```python
from build123d import *

# Parameters (mm, degrees)
SKETCH_1_R          = 18.5
EXTRUDE_1_DEPTH     = 33
SKETCH_2_R          = 18
EXTRUDE_2_DEPTH     = 50
SKETCH_3_R          = 1.6
CUT_EXTRUDE_1_DEPTH = 6
SKETCH_4_R          = 6
EXTRUDE_3_DEPTH     = 6
SKETCH_5_R          = 3
EXTRUDE_4_DEPTH     = 15
CUT_EXTRUDE_START   = -12
CUT_EXTRUDE_2_DEPTH = 12


with BuildPart() as part:
    # 草图1 → 凸台-拉伸1 (new body)
    with BuildSketch(Plane.XY):
        Circle(SKETCH_1_R)
    extrude(amount=EXTRUDE_1_DEPTH)

    # 草图2 → 凸台-拉伸2 (add)
    with BuildSketch(Plane(origin=(0, 0, 0), x_dir=(-1, 0, 0), z_dir=(0, 0, -1))):
        Circle(SKETCH_2_R)
    extrude(amount=EXTRUDE_2_DEPTH)

    # 草图3 → 切除-拉伸1 (cut)
    with BuildSketch(Plane.XY.offset(33)):
        with Locations((-15.5, 0)):
            Circle(SKETCH_3_R)
        with Locations((-7.75, 13.423393759)):
            Circle(SKETCH_3_R)
        with Locations((7.75, 13.423393759)):
            Circle(SKETCH_3_R)
        with Locations((15.5, 0)):
            Circle(SKETCH_3_R)
        with Locations((7.75, -13.423393759)):
            Circle(SKETCH_3_R)
        with Locations((-7.75, -13.423393759)):
            Circle(SKETCH_3_R)
    extrude(amount=-CUT_EXTRUDE_1_DEPTH, mode=Mode.SUBTRACT)

    # 草图4 → 凸台-拉伸3 (add)
    with BuildSketch(Plane.XY.offset(33)):
        with Locations((0, 7)):
            Circle(SKETCH_4_R)
    extrude(amount=EXTRUDE_3_DEPTH)

    # 草图5 → 凸台-拉伸4 (add)
    with BuildSketch(Plane.XY.offset(39)):
        with Locations((0, 7)):
            Circle(SKETCH_5_R)
    extrude(amount=EXTRUDE_4_DEPTH)

    # 草图6 → 切除-拉伸2 (cut)
    with BuildSketch(Plane.XY.offset(54).offset(CUT_EXTRUDE_START)):
        with BuildLine():
            Line((-1.658312395, 9.5), (1.658312395, 9.5))
            ThreePointArc((1.658312395, 9.5), (0, 10), (-1.658312395, 9.5))
        make_face()
    extrude(amount=CUT_EXTRUDE_2_DEPTH, mode=Mode.SUBTRACT)


solid = part.part
```
CAD build for the part. Positions are in the model's coordinates, mm. A direction names the side the tool comes from. Coordinates: 2 decimals unless noted, no trailing zeros. Write each loop counter-clockwise with the first axis right and the second up, starting at its lowest first coordinate (ties: lowest second). Pieces come first, ordered by that corner, then holes. Notation, with made-up numbers: (70, 56.5) -> (74, 56.5) arc R28 cw to (74, 85.5) -> close; hole circle Ø8 at (62.25, 52). An arc over 180 degrees is marked (long way). Use CSV: the item, a comma, the result in double quotes. Start each with the question number.
Item 1: Band-saw the part on C-C, the plane z = -14.5. Write the cut outline in (x, y), plus the area to 3 significant figures.
Item 2: Drop flat-ended pins along their axis: P1, Ø1.7, axis at x = -0.5, z = 47, coming from the +Y side; P2, Ø1.6, axis at x = -16, y = 0, coming from the +Z side; P3, Ø2, axis at x = -4, y = -10.5, coming from the +Z side. Give the stop position or say it passes through.
Item 3: Wall check: probe 1 along Y at (x, z) = (7, 30); probe 2 along Y at (x, z) = (-7.75, 29.85); probe 3 along Z at (x, y) = (-7, -4). Give the ranges that are in metal, low to high.
Item 4: Two-plate mould, pull along X, no slides. Class faces 4 (the flat face through (0, 0, -50)), 5 (the flat face through (8, 13, 27)), 6 (the cylindrical face through (-0.65, 4.07, 46.4)), 7 (the flat face through (-8, -13, 27)): +X half, -X half, draft (parallel to the pull), parting line (faces both ways), or undercut.
Item 5: Band-saw the part on D-D, the plane x = -15.5. Write the cut outline in (y, z).
Item 6: Tool access for faces 1 (the cylindrical face through (-4.01, -18.06, 16.27)), 2 (the cylindrical face through (6.571, 14.505, 30.042)), 3 (the cylindrical face through (2.343, 17.847, -24.65)): list every direction of +Z, -Z, +X, -X, +Y, -Y with a clear straight run to the whole face (end or side of a thin tool).
Item 7: Band-saw the part on A-A, the plane x = 0. Write the cut outline in (y, z), plus the area to 3 significant figures.
Item 8: Band-saw the part on B-B, the plane y = 0. Write the cut outline in (x, z), plus the area to 3 significant figures.
Response values:
1,outline,"circle Ø36 at (0, 0)"
1,area,"1,020 mm2"
2,P1,"stops at y = 9.5"
2,P2,"stops at z = 27"
2,P3,"stops at z = 33"
3,probe 1,"y = -17.12 to -14.84, -12.01 to 12.01, 14.84 to 17.12"
3,probe 2,"y = -16.8 to -15.02, -11.82 to 11.82, 15.02 to 16.8"
3,probe 3,"z = -50 to 33"
4,face 4,"draft"
4,face 5,"undercut"
4,face 6,"parting line"
4,face 7,"undercut"
5,outline,"(-10.1, 0) -> (-9.15, 0) -> (-9.15, -50) -> (9.15, -50) -> (9.15, 0) -> (10.1, 0) -> (10.1, 33) -> (1.6, 33) -> (1.6, 27) -> (-1.6, 27) -> (-1.6, 33) -> (-10.1, 33) -> close"
6,face 1,"+Z, -Z"
6,face 2,"+Z"
6,face 3,"-Z"
7,outline,"(-18.5, 0) -> (-18, 0) -> (-18, -50) -> (18, -50) -> (18, 0) -> (18.5, 0) -> (18.5, 33) -> (13, 33) -> (13, 39) -> (10, 39) -> (10, 42) -> (9.5, 42) -> (9.5, 54) -> (4, 54) -> (4, 39) -> (1, 39) -> (1, 33) -> (-18.5, 33) -> close"
7,area,"3,180 mm2"
8,outline,"(-18.5, 0) -> (-18, 0) -> (-18, -50) -> (18, -50) -> (18, 0) -> (18.5, 0) -> (18.5, 33) -> (17.1, 33) -> (17.1, 27) -> (13.9, 27) -> (13.9, 33) -> (-13.9, 33) -> (-13.9, 27) -> (-17.1, 27) -> (-17.1, 33) -> (-18.5, 33) -> close"
8,area,"2,980 mm2"
